Work out the finished part from the listing and answer in its coordinate system (mm). Face numbers are marked on the shaded views. A direction names the side the tool comes from. Coordinates: 2 decimals unless noted, no trailing zeros. Order: outer loops, then holes, each group sorted by start corner. A loop starts at its lowest first (then second) coordinate and runs counter-clockwise, first axis right, second up. Notation, with made-up numbers: (-6.5, 3.5) -> (6.5, 3.5) arc R20 cw to (6.5, 36.5) -> close; hole circle Ø5 at (27.5, 22.25). An arc over 180 degrees is marked (long way). Use one line per item in the form item = value.
from build123d import *

# Parameters (mm, degrees)
F0_R        = 6.35
F1_DEPTH    = 25.4
F2_W        = 123.3146692741
F2_H        = 9.2131719061
F3_DEPTH    = 44.45
F4_R        = 6.35
F5_R        = 5.08
F6_R        = 5.08
F7_R        = 6.35
F8_R        = 6.35
F9_T1_DEPTH = 31.6918409034
F9_T3_DEPTH = 32.0036689973
F9_T5_DEPTH = 79.9823917725


# Not quite as in the source:
# - a fillet or chamfer that OpenCascade refuses, or shapes differently, is made with other operations: its cross-section is extruded or revolved along the edge and cut away or added


with BuildPart() as f1:
    # F0 (on Top) → F1 (new body)
    with BuildSketch(Plane.XY):
        with BuildLine():
            Line((-38.4631145681, 47.8382077998), (-25.4427038645, 24.9439910361))
            ThreePointArc((-25.4427038645, 24.9439910361), (12.1724359017, 10.8562296523), (7.9763394945, -29.0906918233))
            Line((7.9763394945, -29.0906918233), (35.5361980368, -29.0906918233))
            Line((35.5361980368, -29.0906918233), (46.7120397772, -18.6743740407))
            Line((46.7120397772, -18.6743740407), (14.3780414237, 40.2429682227))
            Line((14.3780414237, 40.2429682227), (-11.6627799835, 47.8382077998))
            Line((-11.6627799835, 47.8382077998), (-38.4631145681, 47.8382077998))
        make_face()
        with Locations((31.4130679807, -17.697843238)):
            Circle(F0_R, mode=Mode.SUBTRACT)
    extrude(amount=F1_DEPTH)

    # F2 (on Front) → F3 (cut, symmetric)
    with BuildSketch(Plane.XZ):
        with Locations((5.399286747, 12.5440859531)):
            Rectangle(F2_W, F2_H)
    extrude(amount=F3_DEPTH, both=True, mode=Mode.SUBTRACT)

    # F4
    f4_edges = [f1.edges().sort_by_distance(p)[0] for p in [
        (14.378041, 40.242968, 21.275336),
    ]]
    fillet(f4_edges, radius=F4_R)

    # F5
    f5_edges = [f1.edges().sort_by_distance(p)[0] for p in [
        (14.378041, 40.242968, 3.96875),
    ]]
    fillet(f5_edges, radius=F5_R)

    # F6
    f6_edges = [f1.edges().sort_by_distance(p)[0] for p in [
        (-11.66278, 47.838208, 12.7),
    ]]
    fillet(f6_edges, radius=F6_R)

    # F7
    f7_edges = [f1.edges().sort_by_distance(p)[0] for p in [
        (7.976339, -29.090692, 21.275336),
        (7.976339, -29.090692, 3.96875),
    ]]
    fillet(f7_edges, radius=F7_R)

    # F8
    f8_edges = [f1.edges().sort_by_distance(p)[0] for p in [
        (35.536198, -29.090692, 3.96875),
        (35.536198, -29.090692, 21.275336),
        (46.71204, -18.674374, 21.275336),
        (46.71204, -18.674374, 3.96875),
    ]]
    fillet(f8_edges, radius=F8_R)

    # F9: fillet of radius 6.35 on 3 edges, made by hand

    # F9_s2 → F9_t1 (cut)
    with BuildSketch(Plane.XY.offset(-11.8771704517)):
        with BuildLine():
            ThreePointArc((-21.2123797216, 25.95187937), (-24.9938313602, 26.4760275688), (-27.791358986, 29.0737086524))
            Line((-27.791358986, 29.0737086524), (-25.4427038645, 24.9439910361))
            ThreePointArc((-25.4427038645, 24.9439910361), (-23.3442549108, 25.5180837534), (-21.2123797216, 25.95187937))
        make_face()
    extrude(amount=F9_T1_DEPTH, mode=Mode.SUBTRACT)

    # F9_s4 → F9_t3 (cut)
    with BuildSketch(Plane.XY.offset(5.2735014544)):
        with BuildLine():
            ThreePointArc((-27.791358986, 29.0737086524), (-24.9938313602, 26.4760275688), (-21.2123797216, 25.95187937))
            ThreePointArc((-21.2123797216, 25.95187937), (-23.3442549108, 25.5180837534), (-25.4427038645, 24.9439910361))
            Line((-25.4427038645, 24.9439910361), (-27.791358986, 29.0737086524))
        make_face()
    extrude(amount=F9_T3_DEPTH, mode=Mode.SUBTRACT)

    # F9_s6 → F9_t5 (cut)
    with BuildSketch(Plane.XY.offset(-27.2911958862)):
        with BuildLine():
            ThreePointArc((-33.0664077304, 38.3490005109), (-33.0355553369, 44.6810539999), (-27.5466362136, 47.8382077998))
            Line((-27.5466362136, 47.8382077998), (-38.4631145681, 47.8382077998))
            Line((-38.4631145681, 47.8382077998), (-33.0664077304, 38.3490005109))
        make_face()
    extrude(amount=F9_T5_DEPTH, mode=Mode.SUBTRACT)


solid = f1.part
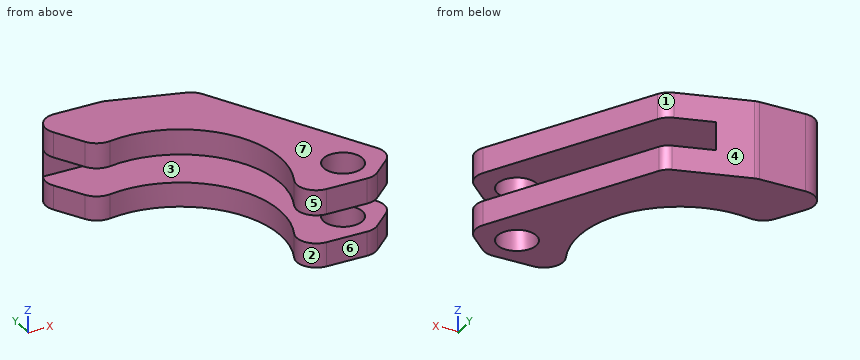
(1) Section A-A on y = 17.5 is taken. Write down the section's boundary in (x, z) (1 decimal), plus the area to 3 significant figures.
Data:
outline = (6.7, 0) -> (26.9, 0) -> (26.9, 7.9) -> (6.7, 7.9) -> close; (6.7, 17.2) -> (26.9, 17.2) -> (26.9, 25.4) -> (6.7, 25.4) -> close
area = 326 mm²
(2) Each of these flat-tipped pins is pushed along its axis until it touches: P1, Ø2, axis at y = -13.5, z = 8, coming from the +X side; P2, Ø1.5, axis at y = 28, z = 21.5, coming from the -X side; P3, Ø7.5, axis at x = -13, z = 12.5, coming from the -Y side. Where does it stop, or does it pass through?
Data:
P1 = 44.42
P2 = -27.59
P3 = 44.45
(3) Straight lines are drawn through the part: line 1 along Z through (x, y) = (17, 6); line 2 along Y through (x, z) = (20.5, 4.25); line 3 along Y through (x, z) = (-16, 8.5). For each, find the intervals that lie inside material, in ascending order.
Data:
line_1 = 0 to 7.94, 17.15 to 25.4
line_2 = -29.09 to 29.09
line_3 = 44.45 to 47.84
(4) Which of the six approach directions +Z, -Z, +X, -X, +Y, -Y give full straight-line access (tool end or side, diameter ignored) to the marked faces 1, 2 and 3?
Data:
face_1 = +Z, +X, +Y
face_2 = +Z, -Z, -X
face_3 = +X, -X, -Y
(5) The mould has two halves that part along Y. Classify the marked faces 4, 5, 6 and 7: released by +Y, released by -Y, zero draft, split by the parting line, or undercut.
Data:
face_4 = released by +Y
face_5 = undercut
face_6 = released by -Y
face_7 = zero draft
(6) Section C-C on x = 9.5 is taken. Write down the section's boundary in (y, z).
Data:
outline = (14.57, 0) -> (41.67, 0) -> (41.67, 7.94) -> (14.57, 7.94) -> close; (14.57, 17.15) -> (41.67, 17.15) -> (41.67, 25.4) -> (14.57, 25.4) -> close
